```python
from build123d import *
from build123d.topology import SkipClean

# Parameters (mm, degrees)
SKETCH_1_R          = 2.6
SKETCH_1_R_2        = 4
EXTRUDE_1_DEPTH     = 4
EXTRUDE_START       = 4
SKETCH_2_R          = 12.9
SKETCH_2_R_2        = 4
EXTRUDE_2_DEPTH     = 4
EXTRUDE_START_2     = 3.5
SKETCH_3_R          = 6.1
SKETCH_3_R_2        = 4
EXTRUDE_3_DEPTH     = 3.5
SKETCH_6_R          = 1
CUT_EXTRUDE_1_DEPTH = 10
SKETCH_7_R          = 1
CUT_EXTRUDE_2_DEPTH = 10


with BuildPart() as part:
    # 草图1 → 凸台-拉伸1 (new body)
    with BuildSketch(Plane(origin=(0, 0, 0), x_dir=(1, 0, 0), z_dir=(0, 1, 0))):
        with BuildLine():
            Line((-20.70972973, -5.145589813), (-5.09027027, -11.853233676))
            ThreePointArc((-5.09027027, -11.853233676), (0, -12.9), (5.09027027, -11.853233676))
            Line((5.09027027, -11.853233676), (20.70972973, -5.145589813))
            ThreePointArc((20.70972973, -5.145589813), (24.1, 0), (20.70972973, 5.145589813))
            Line((20.70972973, 5.145589813), (5.09027027, 11.853233676))
            ThreePointArc((5.09027027, 11.853233676), (0, 12.9), (-5.09027027, 11.853233676))
            Line((-5.09027027, 11.853233676), (-20.70972973, 5.145589813))
            ThreePointArc((-20.70972973, 5.145589813), (-24.1, 0), (-20.70972973, -5.145589813))
        make_face()
        with Locations(Location((-18.5, 0, 0), (0, 0, 270))):
            Circle(SKETCH_1_R, mode=Mode.SUBTRACT)
        with Locations(Location((18.5, 0, 0), (0, 0, 90))):
            Circle(SKETCH_1_R, mode=Mode.SUBTRACT)
        with Locations(Location((0, 0, 0), (0, 0, 270))):
            Circle(SKETCH_1_R_2, mode=Mode.SUBTRACT)
    extrude(amount=EXTRUDE_1_DEPTH)

    # 草图2 → 凸台-拉伸2 (add)
    with SkipClean():  # the faces are left unmerged after this step: merging them gives an invalid solid
        with BuildSketch(Plane.XZ.offset(EXTRUDE_START)):
            with Locations(Location((0, 0, 0), (0, 0, 270))):
                Circle(SKETCH_2_R)
            with Locations(Location((0, 0, 0), (0, 0, 270))):
                Circle(SKETCH_2_R_2, mode=Mode.SUBTRACT)
        extrude(amount=-EXTRUDE_2_DEPTH)

    # 草图3 → 凸台-拉伸3 (add)
    with SkipClean():  # the faces are left unmerged after this step: merging them gives an invalid solid
        with BuildSketch(Plane.XZ.offset(4).offset(EXTRUDE_START_2)):
            with Locations(Location((0, 0, 0), (0, 0, 270))):
                Circle(SKETCH_3_R)
            with Locations(Location((0, 0, 0), (0, 0, 270))):
                Circle(SKETCH_3_R_2, mode=Mode.SUBTRACT)
        extrude(amount=-EXTRUDE_3_DEPTH)

    # 草图6 → 切除-拉伸1 (cut)
    with SkipClean():  # the faces are left unmerged after this step: merging them gives an invalid solid
        with BuildSketch(Plane.XY):
            with Locations(Location((0, -5.75, 0), (0, 0, 90))):
                Circle(SKETCH_6_R)
        extrude(amount=-CUT_EXTRUDE_1_DEPTH, mode=Mode.SUBTRACT)

    # 草图7 → 切除-拉伸2 (cut)
    with SkipClean():  # the faces are left unmerged after this step: merging them gives an invalid solid
        with BuildSketch(Plane(origin=(0, 0, 0), x_dir=(0, 0, -1), z_dir=(1, 0, 0))):
            with Locations((0, -5.75)):
                Circle(SKETCH_7_R)
        extrude(amount=-CUT_EXTRUDE_2_DEPTH, mode=Mode.SUBTRACT)


solid = part.part
```
Could you check a few things on this model? Use its own coordinates, in mm. A direction names the side the tool comes from. Give positions to 0.01 mm unless a question says otherwise; leave off trailing zeros. Order: outer loops, then holes, each group sorted by start corner. A loop starts at its lowest first (then second) coordinate and runs counter-clockwise, first axis right, second up.
Q1. I'm going to push flat-ended pins straight in: P1, Ø4, axis at x = 4.5, y = 2.5, coming from the +Z side; P2, Ø1, axis at x = -10, y = 0.5, coming from the -Z side; P3, Ø3, axis at x = -5.5, z = 6.5, coming from the -Y side. Where does each tip first touch, or does it pass through?
Q2. If I drill on line 1 along Y through (x, z) = (-5.55, 0); line 2 along Z through (x, y) = (0, -1.25); line 3 along X through (y, z) = (-4.95, 0), over which ranges is the centre line in solid material (lowest first)?
Q3. Suppose I cut it at A-A, the plane z = 0. Write out the boundary of the cut face in (x, y).
Q4. For faces 4 (the cylindrical face through (-3.71, -5.77, 4.84)), 5 (the flat face through (-12.791, 1.972, -8.546)), which set-ups out of +Z, -Z, +X, -X, +Y, -Y let a thin tool reach every point of the face, with its end or its side?
Q5. We'd pull the mould along Z, two halves only. Please class faces 1 (the flat face through (13.01, 1.97, -8.45)), 2 (the cylindrical face through (-4.97, -5.45, -0.954)), 3 (the cylindrical face through (-0.04, -6.75, -4.97)): +Z half, -Z half, draft (parallel to the pull), parting line (faces both ways), or undercut.
Q6. Suppose I cut it at D-D, the plane y = -5.75. Write out the boundary of the cut face in (x, z), and give its area (3 significant figures).
Q7. Suppose I cut it at C-C, the plane y = 3. Write out the boundary of the cut face in (x, z).
Q8. Suppose I cut it at B-B, the plane x = -18.5. Write out the boundary of the cut face in (y, z).
Solution:
1. P1: stops at z = 12.66
1. P2: stops at z = -9.96
1. P3: stops at y = -4
2. line 1: y = -7.5 to -6.75, -4.75 to 4
2. line 2: z = -12.9 to -4, 4 to 12.9
2. line 3: x = 4 to 6.1
3. outline: (-24.1, 0) - (-21.1, 0) - (-21.1, 4) - (-24.1, 4) - close; (-15.9, 0) - (-12.9, 0) - (-12.9, -4) - (-6.1, -4) - (-6.1, -4.75) - (-4, -4.75) - (-4, 4) - (-15.9, 4) - close; (-6.1, -7.5) - (-4, -7.5) - (-4, -6.75) - (-6.1, -6.75) - close; (4, -7.5) - (6.1, -7.5) - (6.1, -4) - (12.9, -4) - (12.9, 0) - (15.9, 0) - (15.9, 4) - (4, 4) - close; (21.1, 0) - (24.1, 0) - (24.1, 4) - (21.1, 4) - close
4. face 4: -Y
4. face 5: -Z, -X, +Y, -Y
5. face 1: -Z half
5. face 2: undercut
5. face 3: draft
6. outline: (-6.02, -1) arc R6.1 ccw to (-1, -6.02) - (-1, -3.87) arc R4 cw to (-3.87, -1) - close; (-6.02, 1) - (-3.87, 1) arc R4 cw (long way) to (1, -3.87) - (1, -6.02) arc R6.1 ccw (long way) to start
6. area: 58.2 mm2
7. outline: (-20.71, -5.15) - (-5.09, -11.85) arc R12.9 ccw to (5.09, -11.85) - (20.71, -5.15) arc R5.6 ccw to (20.71, 5.15) - (5.09, 11.85) arc R12.9 ccw to (-5.09, 11.85) - (-20.71, 5.15) arc R5.6 ccw to start; hole circle Ø5.2 at (-18.5, 0); hole circle Ø8 at (0, 0); hole circle Ø5.2 at (18.5, 0)
8. outline: (0, -6.09) - (4, -6.09) - (4, -2.6) - (0, -2.6) - close; (0, 2.6) - (4, 2.6) - (4, 6.09) - (0, 6.09) - close
